```python
from build123d import *

# Parameters (mm, degrees)
SKETCH_W        = 50
SKETCH_H        = 80
PAD_DEPTH       = 40
SKETCH001_W     = 42
SKETCH001_H     = 72
POCKET_DEPTH    = 36
SKETCH002_W     = 42
SKETCH002_H     = 10
PAD001_DEPTH    = 18
SKETCH003_R     = 13
POCKET001_DEPTH = 30
SKETCH004_W     = 42
SKETCH004_H     = 10
PAD002_DEPTH    = 18
SKETCH005_R     = 13
POCKET002_DEPTH = 10
PAD003_DEPTH    = 5
PAD004_DEPTH    = 5
SKETCH008_R     = 5
POCKET003_DEPTH = 19
POCKET004_DEPTH = 5
SKETCH010_R     = 4
POCKET005_DEPTH = 5
SKETCH011_W     = 15
SKETCH011_H     = 5
PAD005_DEPTH    = 15
SKETCH012_W     = 15
SKETCH012_H     = 5
PAD006_DEPTH    = 15
SKETCH013_R     = 2.5
POCKET006_DEPTH = 5
FILLET_R        = 6
FILLET001_R     = 6
FILLET002_R     = 6
SKETCH014_R     = 1.6
POCKET007_DEPTH = 95.001


with BuildPart() as part:
    # Sketch → Pad (new body)
    with BuildSketch(Plane.XY):
        with Locations((-25, 40)):
            Rectangle(SKETCH_W, SKETCH_H)
    extrude(amount=PAD_DEPTH)

    # Sketch001 (on Face6 of Pad) → Pocket (cut)
    with BuildSketch(Plane.XY.offset(40)):
        with Locations((-25, 40)):
            Rectangle(SKETCH001_W, SKETCH001_H)
    extrude(amount=-POCKET_DEPTH, mode=Mode.SUBTRACT)

    # Sketch002 (on Face11 of Pocket) → Pad001 (join)
    with BuildSketch(Plane.XY.offset(4)):
        with Locations((-25, 34)):
            Rectangle(SKETCH002_W, SKETCH002_H)
    extrude(amount=PAD001_DEPTH)

    # Sketch003 (on Face13 of Pad001) → Pocket001 (cut)
    with BuildSketch(Plane.XZ.offset(-29)):
        with Locations((-25, 22)):
            Circle(SKETCH003_R)
    extrude(amount=-POCKET001_DEPTH, mode=Mode.SUBTRACT)

    # Sketch004 (on Face11 of Pocket001) → Pad002 (join)
    with BuildSketch(Plane.XY.offset(4)):
        with Locations((-25, 49)):
            Rectangle(SKETCH004_W, SKETCH004_H)
    extrude(amount=PAD002_DEPTH)

    # Sketch005 (on Face17 of Pad002) → Pocket002 (cut)
    with BuildSketch(Plane.XZ.offset(-44)):
        with Locations((-25, 22)):
            Circle(SKETCH005_R)
    extrude(amount=-POCKET002_DEPTH, mode=Mode.SUBTRACT)

    # Sketch006 (on Face17 of Pocket002) → Pad003 (join)
    with BuildSketch(Plane.XZ.offset(-44)):
        with BuildLine():
            ThreePointArc((-39, 17), (-41, 19), (-43, 17))
            Line((-43, 17), (-43, 12))
            ThreePointArc((-43, 12), (-41, 10), (-39, 12))
            Line((-39, 17), (-39, 12))
        make_face()
        with BuildLine():
            ThreePointArc((-7, 17), (-9, 19), (-11, 17))
            Line((-11, 17), (-11, 12))
            ThreePointArc((-11, 12), (-9, 10), (-7, 12))
            Line((-7, 17), (-7, 12))
        make_face()
    extrude(amount=PAD003_DEPTH)

    # Sketch007 (on Face13 of Pad003) → Pad004 (join)
    with BuildSketch(Plane.XZ.offset(-29)):
        with BuildLine():
            ThreePointArc((-38, 22), (-25, 9), (-12, 22))
            Line((-16, 22), (-12, 22))
            ThreePointArc((-34, 22), (-25, 13), (-16, 22))
            Line((-38, 22), (-34, 22))
        make_face()
    extrude(amount=-PAD004_DEPTH)

    # Sketch008 (on Face2 of Pad004) → Pocket003 (cut)
    with BuildSketch(Plane.YZ):
        with Locations((29, 22)):
            Circle(SKETCH008_R)
    extrude(amount=-POCKET003_DEPTH, mode=Mode.SUBTRACT)

    # Sketch009 (on Face6 of Pocket003) → Pocket004 (cut)
    with BuildSketch(Plane(origin=(0, 80, 0), x_dir=(-1, 0, 0), z_dir=(0, 1, 0))):
        with BuildLine():
            ThreePointArc((22.5, 23.5), (21, 22), (22.5, 20.5))
            Line((22.5, 20.5), (27.5, 20.5))
            ThreePointArc((27.5, 20.5), (29, 22), (27.5, 23.5))
            Line((22.5, 23.5), (27.5, 23.5))
        make_face()
    extrude(amount=-POCKET004_DEPTH, mode=Mode.SUBTRACT)

    # Sketch010 (on Face1 of Pocket004) → Pocket005 (cut)
    with BuildSketch(Plane.XZ):
        with Locations((-25, 22)):
            Circle(SKETCH010_R)
    extrude(amount=-POCKET005_DEPTH, mode=Mode.SUBTRACT)

    # Sketch011 (on Face7 of Pocket005) → Pad005 (join)
    with BuildSketch(Plane(origin=(0, 80, 0), x_dir=(-1, 0, 0), z_dir=(0, 1, 0))):
        with Locations((25, 2.5)):
            Rectangle(SKETCH011_W, SKETCH011_H)
    extrude(amount=PAD005_DEPTH)

    # Sketch012 (on Face1 of Pad005) → Pad006 (join)
    with BuildSketch(Plane.XZ):
        with Locations((-25, 2.5)):
            Rectangle(SKETCH012_W, SKETCH012_H)
    extrude(amount=PAD006_DEPTH)

    # Sketch013 (on Face20 of Pad006) → Pocket006 (cut)
    with BuildSketch(Plane.XY.offset(5)):
        with Locations((-25, 88.385622)):
            Circle(SKETCH013_R)
        with Locations((-25, -8.385622)):
            Circle(SKETCH013_R)
    extrude(amount=-POCKET006_DEPTH, mode=Mode.SUBTRACT)

    # Fillet
    fillet_edges = [part.edges().sort_by_distance(p)[0] for p in [
        (-32.5, -15, 2.5),
        (-17.5, -15, 2.5),
        (-32.5, 95, 2.5),
        (-17.5, 95, 2.5),
    ]]
    fillet(fillet_edges, radius=FILLET_R)

    # Fillet001
    fillet001_edges = [part.edges().sort_by_distance(p)[0] for p in [
        (-46, 16.5, 4),
        (-25, 4, 4),
        (-4, 16.5, 4),
        (-25, 29, 4),
        (-46, 4, 22),
        (-46, 76, 22),
        (-4, 76, 22),
        (-4, 4, 22),
    ]]
    fillet(fillet001_edges, radius=FILLET001_R)

    # Fillet002
    fillet002_edges = [part.edges().sort_by_distance(p)[0] for p in [
        (0, 0, 20),
        (-50, 0, 20),
        (-50, 80, 20),
        (0, 80, 20),
    ]]
    fillet(fillet002_edges, radius=FILLET002_R)

    # Sketch014 (on Face9 of Fillet002) → Pocket007 (cut, through all)
    with BuildSketch(Plane(origin=(0, 80, 0), x_dir=(-1, 0, 0), z_dir=(0, 1, 0))):
        with Locations((25, 32)):
            Circle(SKETCH014_R)
    extrude(amount=-POCKET007_DEPTH, mode=Mode.SUBTRACT)


solid = part.part
```
The listing builds one solid part. Answer for the finished solid, in the listing's coordinates (mm). A direction names the side the tool comes from. Coordinates: 2 decimals unless noted, no trailing zeros. Write each loop counter-clockwise with the first axis right and the second up, starting at its lowest first coordinate (ties: lowest second). Pieces come first, ordered by that corner, then holes. Notation, with made-up numbers: (23.25, 67.5) - (49.25, 67.5) arc R32 ccw to (49.25, 99.5) - close; hole circle Ø2 at (34.25, 18). An arc over 180 degrees is marked (long way). Return JSON: item names as keys, results as strings. Group by question number.
Q1. Find the intervals of material crossed by line 1 along Y through (x, z) = (-25, 3.9); line 2 along Y through (x, z) = (-40.5, 19.5); line 3 along Z through (x, y) = (-25, 2), in increasing order. Write a range as [from, to].
Q2. The part is cut by section D-D on x = -41.5. Write down the section's boundary in (y, z).
Q3. The part is cut by section C-C on x = -25. State how many separate pieces and enclosed holes the cut face has, and give its area (3 significant figures).
Q4. Which of the six approach directions +Z, -Z, +X, -X, +Y, -Y give full straight-line access (tool end or side, diameter ignored) to faces 1 (the flat face through (-42, 49, 22)), 2 (the cylindrical face through (-21, 78, 22)), 3 (the cylindrical face through (-26.98, -9.91, 2.54))?
Q5. The part is cut by section A-A on z = 32. Write down the section's boundary in (x, y), and give its area (3 significant figures).
Q6. The part is cut by section B-B on y = 61.5. Write down the section's boundary in (x, z), and give its area (3 significant figures).
Q7. For a pull along Z with two mould halves and no side action, classify faces 4 (the cylindrical face through (-29, 78, 22)), 5 (the flat face through (-25.1, -5.7, 5)), 6 (the flat face through (-29, 0, 20)) as +Z half, -Z half, draft (parallel to the pull), parting line (faces both ways), or undercut.
Q8. Flat-ended cylindrical pins translate along their axes: pin 1 Ø14.5 at (x, z) = (-29, 8.5) entering from -Y; pin 2 Ø3 at (x, y) = (-37.5, 34.5) entering from +Z; pin 3 Ø12 at (x, y) = (-31.5, 13.5) entering from +Z; pin 4 Ø3 at (x, y) = (-16, 69) entering from +Z. Find the tip coordinate at first contact, or state that the pin passes through.
Evaluation:
{
 "1": {"line 1": "y = [-15, -10.89], [-5.89, 85.89], [90.89, 95]", "line 2": "y = [0, 4.02], [29, 39], [44, 54], [75.98, 80]", "line 3": "z = [0, 18], [26, 30.4], [33.6, 40]"},
 "2": {"outline": "(0, 0) - (80, 0) - (80, 40) - (75.81, 40) - (75.81, 4) - (54, 4) - (54, 22) - (44, 22) - (44, 18.94) - (39, 18.94) - (39, 22) - (29, 22) - (29, 10) arc R6 cw to (24.5, 4.19) - (10, 4.19) arc R5.81 cw to (4.19, 10) - (4.19, 40) - (0, 40) - close; hole (39, 4) - (44, 4) - (44, 10.06) - (39, 10.06) - close"},
 "3": {"separate pieces": "7", "enclosed holes": "0", "area": "774 mm2"},
 "4": {"face 1": "+Z", "face 2": "+Y, -Y", "face 3": "+Z, -Z"},
 "5": {"outline": "(-50, 6) arc R6 ccw to (-44, 0) - (-26.6, 0) - (-26.6, 4) - (-40, 4) arc R6 cw to (-46, 10) - (-46, 70) arc R6 cw to (-40, 76) - (-26.6, 76) - (-26.6, 80) - (-44, 80) arc R6 ccw to (-50, 74) - close; (-23.4, 0) - (-6, 0) arc R6 ccw to (0, 6) - (0, 74) arc R6 ccw to (-6, 80) - (-23.4, 80) - (-23.4, 76) - (-10, 76) arc R6 cw to (-4, 70) - (-4, 10) arc R6 cw to (-10, 4) - (-23.4, 4) - close", "area": "950 mm2"},
 "6": {"outline": "(-50, 0) - (0, 0) - (0, 40) - (-4, 40) - (-4, 4) - (-46, 4) - (-46, 40) - (-50, 40) - close", "area": "488 mm2"},
 "7": {"face 4": "undercut", "face 5": "+Z half", "face 6": "draft"},
 "8": {"pin 1": "stops at y = -15", "pin 2": "stops at z = 22", "pin 3": "stops at z = 4.55", "pin 4": "stops at z = 4"}
}
